The model under review builds one solid part; all positions refer to its coordinate system, in mm. Coordinates: 2 decimals unless noted, no trailing zeros. Order: outer loops, then holes, each group sorted by start corner. A loop starts at its lowest first (then second) coordinate and runs counter-clockwise, first axis right, second up. Notation, with made-up numbers: (69.25, -36) - (110.25, -36) arc R20 ccw to (110.25, 1) - close; hole circle Ø5 at (64, -25). An arc over 180 degrees is marked (long way). Answer in a Markdown table with one row per item.
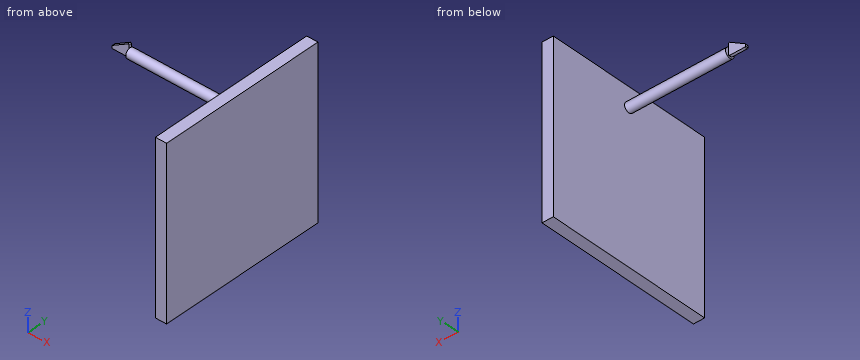
```python
from build123d import *

# Parameters (mm, degrees)
F1_DEPTH = 3.175
F2_R     = 11.049
F3_DEPTH = 228.6
F4_W     = 381
F4_H     = 381
F5_DEPTH = 25.4


with BuildPart() as f1:
    # F0 (on Front) → F1 (new body, symmetric)
    with BuildSketch(Plane.XZ):
        with BuildLine():
            Line((0, -6.223), (0, 18.5326917232))
            ThreePointArc((0, 18.5326917232), (-0.7698692632, 19.8570265871), (-2.3016572596, 19.843350026))
            Line((-2.3016572596, 19.843350026), (-37.3536572596, -0.954169974))
            ThreePointArc((-37.3536572596, -0.954169974), (-37.9003348639, -1.51069754), (-38.1, -2.2648282768))
            Line((-38.1, -2.2648282768), (-38.1, -6.223))
            ThreePointArc((-38.1, -6.223), (-37.6536307345, -7.3006307345), (-36.576, -7.747))
            Line((-36.576, -7.747), (-1.524, -7.747))
            ThreePointArc((-1.524, -7.747), (-0.4463692655, -7.3006307345), (0, -6.223))
        make_face()
    extrude(amount=F1_DEPTH, both=True)

    # F2 (on Right) → F3 (join)
    with BuildSketch(Plane.YZ):
        Circle(F2_R)
    extrude(amount=F3_DEPTH)

    # F4 (on face) → F5 (join)
    with BuildSketch(Plane.YZ.offset(228.6)):
        with Locations((0, -146.05)):
            Rectangle(F4_W, F4_H)
    extrude(amount=F5_DEPTH)


solid = f1.part
```
Item 1: We need section B-B, the plane y = 58. Write out the cut boundary in (x, z).
Check values:
| item | result |
|---|---|
| outline | (228.6, -336.55) - (254, -336.55) - (254, 44.45) - (228.6, 44.45) - close |
Item 2: Clearance check with flat-ended pins moving along their axes: pin 1 Ø8.5 at (x, z) = (-17, 6.5) entering from +Y (3 decimals); pin 2 Ø7 at (x, y) = (-23, 1) entering from -Z; pin 3 Ø8 at (y, z) = (-25.5, -31.5) entering from -X. State where each tip first meets the part, or that it passes through.
Check values:
| item | result |
|---|---|
| pin 1 | y = 3.175 |
| pin 2 | z = -7.75 |
| pin 3 | x = 228.6 |
Item 3: We need section C-C, the plane z = -193.5. Write out the cut boundary in (x, y).
Check values:
| item | result |
|---|---|
| outline | (228.6, -190.5) - (254, -190.5) - (254, 190.5) - (228.6, 190.5) - close |
Item 4: We need section A-A, the plane x = 99.5. Write out the cut boundary in (y, z), then the cut area to 3 significant figures.
Check values:
| item | result |
|---|---|
| outline | circle Ø22.1 at (0, 0) |
| area | 384 mm^2 |
Item 5: To check wall thickness, follow line 1 (X direction, y = -127.5, z = -279.5); line 2 (Y direction, x = 12.5, z = 4). State the ranges of each line that lie inside material, in increasing order. Write a range as from..to.
Check values:
| item | result |
|---|---|
| line 1 | 228.6..254 |
| line 2 | -10.3..10.3 |
